```python
from build123d import *

# Parameters (mm, degrees)
SKETCH1_W           = 66
SKETCH1_H           = 70
BOSS_EXTRUDE1_DEPTH = 2
SKETCH2_W           = 2
SKETCH2_H           = 20
BOSS_EXTRUDE2_DEPTH = 2
SKETCH3_W           = 20
SKETCH3_H           = 2
BOSS_EXTRUDE3_DEPTH = 2


with BuildPart() as part:
    # Sketch1 → Boss-Extrude1 (new body)
    with BuildSketch(Plane.XY):
        Rectangle(SKETCH1_W, SKETCH1_H)
    extrude(amount=BOSS_EXTRUDE1_DEPTH)

    # Sketch2 → Boss-Extrude2 (add)
    with BuildSketch(Plane(origin=(0, 0, 0), x_dir=(-1, 0, 0), z_dir=(0, 0, -1))):
        with Locations((34, -15)):
            Rectangle(SKETCH2_W, SKETCH2_H)
        with Locations((34, 15)):
            Rectangle(SKETCH2_W, SKETCH2_H)
        with Locations((-34, -15)):
            Rectangle(SKETCH2_W, SKETCH2_H)
        with Locations((-34, 15)):
            Rectangle(SKETCH2_W, SKETCH2_H)
    extrude(amount=-BOSS_EXTRUDE2_DEPTH)

    # Sketch3 → Boss-Extrude3 (add)
    with BuildSketch(Plane(origin=(0, 0, 0), x_dir=(-1, 0, 0), z_dir=(0, 0, -1))):
        with Locations((-15, 36)):
            Rectangle(SKETCH3_W, SKETCH3_H)
        with Locations((15, 36)):
            Rectangle(SKETCH3_W, SKETCH3_H)
        with Locations((-15, -36)):
            Rectangle(SKETCH3_W, SKETCH3_H)
        with Locations((15, -36)):
            Rectangle(SKETCH3_W, SKETCH3_H)
    extrude(amount=-BOSS_EXTRUDE3_DEPTH)


solid = part.part
```
Part model, mm, in its own coordinate system. A direction names the side the tool comes from. Round coordinates to 2 decimals unless told otherwise and drop trailing zeros. Loops run counter-clockwise (first coordinate to the right, second up) from the corner with the lowest first, then second, coordinate; pieces in that order, holes last. Notation, with made-up numbers: (-7, 14) -> (20, 14) arc R28 cw to (20, 35) -> close; hole circle Ø7 at (53, 70.5). An arc over 180 degrees is marked (long way). Use one line per item in the form item = value. Start each with the question number.
Item 1: Drill centre lines: line 1 along Y through (x, z) = (1, 0.5); line 2 along X through (y, z) = (-26.5, 1.25). Where is each one in solid material? Low to high.
Item 2: Drop flat-ended pins along their axis: pin 1 Ø0.6 at (x, z) = (34.5, 1) entering from -Y; pin 2 Ø1 at (y, z) = (-31.5, 1.5) entering from +X; pin 3 Ø1 at (y, z) = (-36, 1) entering from -X. Give the stop position or say it passes through.
Item 3: Tool access for faces 5 (the flat face through (-34, -25, 1)), 6 (the flat face through (34, -5, 1)), 7 (the flat face through (34, 25, 1)), 8 (the flat face through (-33, 30, 1)): list every direction of +Z, -Z, +X, -X, +Y, -Y with a clear straight run to the whole face (end or side of a thin tool).
Item 4: Two-plate mould, pull along X, no slides. Class faces 1 (the flat face through (-15, 37, 1)), 2 (the flat face through (5, -36, 1)), 3 (the flat face through (-35, 15, 1)), 4 (the flat face through (5, 36, 1)): released by +X, released by -X, zero draft, split by the parting line, or undercut.
Item 5: Band-saw the part on A-A (y = -27). List the corners of the cut face in (x, z).
Data:
q1.line_1 = -35 to 35
q1.line_2 = -33 to 33
q2.pin_1 = -25
q2.pin_2 = 33
q2.pin_3 = -25
q3.face_5 = +Z, -Z, -X, -Y
q3.face_6 = +Z, -Z, +X
q3.face_7 = +Z, -Z, +X, +Y
q3.face_8 = +Z, -Z, -X, +Y
q4.face_1 = zero draft
q4.face_2 = undercut
q4.face_3 = released by -X
q4.face_4 = undercut
q5.outline = (-33, 0) -> (33, 0) -> (33, 2) -> (-33, 2) -> close
